Geometry check sheet. Reference: drawing and pictorial views, mm from the part's lowest x, y, z. Give positions to 0.01 mm unless a question says otherwise; leave off trailing zeros. Loops run counter-clockwise (first coordinate to the right, second up) from the corner with the lowest first, then second, coordinate; pieces in that order, holes last. Notation, with made-up numbers: (35.5, 86.5) - (47.5, 86.5) arc R30 cw to (47.5, 120.5) - close; hole circle Ø6 at (40, -8). An arc over 180 degrees is marked (long way). Answer in a Markdown table with one row per item. Add a question column.
(1) Thickness scan on L1, parallel to X at y = 1.15, z = 78; L2, parallel to X at y = 0.5, z = 30.5; L3, parallel to X at y = 1.25, z = 66. Record the ranges inside material, lowest first.
(2) Sectioned sample at A-A on z = 54.8. Enter the section's corners in (x, y), then the cut area to 3 significant figures.
(3) Sectioned sample at B-B on x = 109.8. Enter the section's corners in (y, z).
(4) Sectioned sample at C-C on z = 32.3. Enter the section's corners in (x, y), then the cut area to 3 significant figures.
(5) Go/stop test with flat-tipped pins: P1, Ø8, axis at x = 14.8, z = 72.8, coming from the -Y side; P2, Ø1.5, axis at x = 4.5, y = 1.5, coming from the -Z side; P3, Ø0.9, axis at x = 3.5, y = 1, coming from the +Z side. Record where each tip stops, or that it passes through.
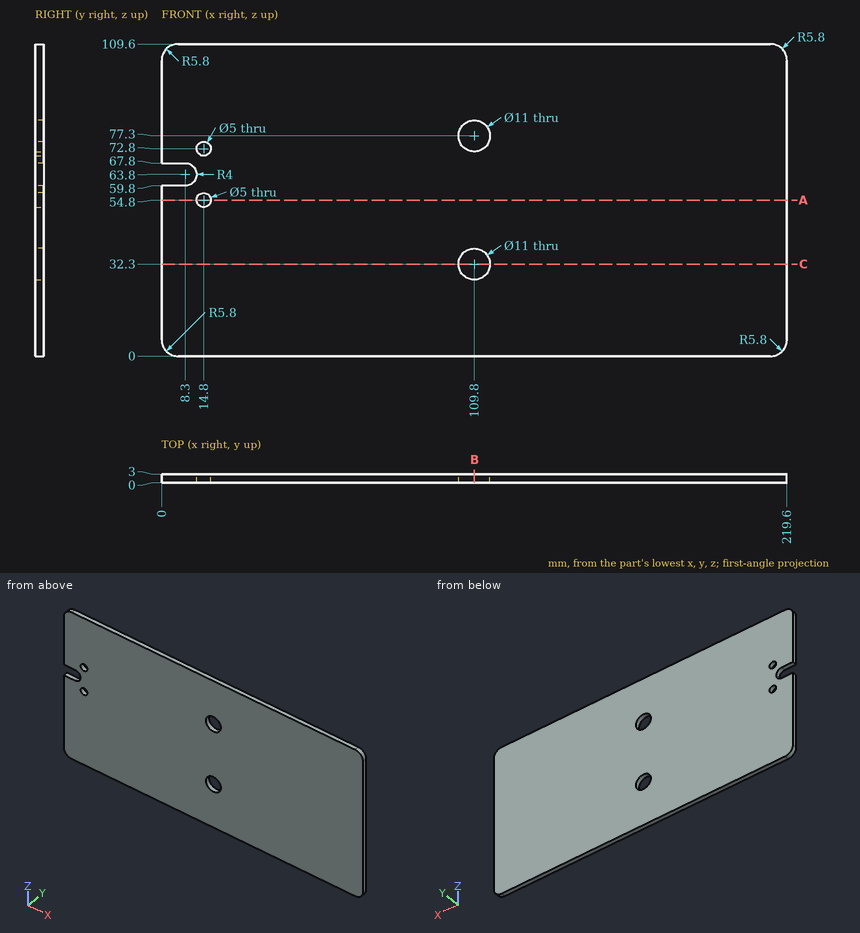
Reply:
| question | item | result |
|---|---|---|
| 1 | L1 | 0 to 104.34, 115.26 to 219.6 |
| 1 | L2 | 0 to 104.6, 115 to 219.6 |
| 1 | L3 | 11.64 to 219.6 |
| 2 | outline | (0, 0) - (12.3, 0) - (12.3, 3) - (0, 3) - close; (17.3, 0) - (219.6, 0) - (219.6, 3) - (17.3, 3) - close |
| 2 | area | 644 mm^2 |
| 3 | outline | (0, 0) - (3, 0) - (3, 26.8) - (0, 26.8) - close; (0, 37.8) - (3, 37.8) - (3, 71.8) - (0, 71.8) - close; (0, 82.8) - (3, 82.8) - (3, 109.6) - (0, 109.6) - close |
| 4 | outline | (0, 0) - (104.3, 0) - (104.3, 3) - (0, 3) - close; (115.3, 0) - (219.6, 0) - (219.6, 3) - (115.3, 3) - close |
| 4 | area | 626 mm^2 |
| 5 | P1 | y = 0 |
| 5 | P2 | z = 0.03 |
| 5 | P3 | z = 109.3 |
